Geometry: see drawing. Coordinates: mm, zero at the bounding-box minimum. A direction names the side the tool comes from. Round coordinates to 2 decimals unless told otherwise and drop trailing zeros. Write each loop counter-clockwise with the first axis right and the second up, starting at its lowest first coordinate (ties: lowest second). Pieces come first, ordered by that corner, then holes. Notation, with made-up numbers: (66, 80.5) -> (96, 80.5) arc R30 cw to (96, 108.5) -> close; hole circle Ø4 at (0, 56). An arc over 180 degrees is marked (long way). Write item = value, one per line.
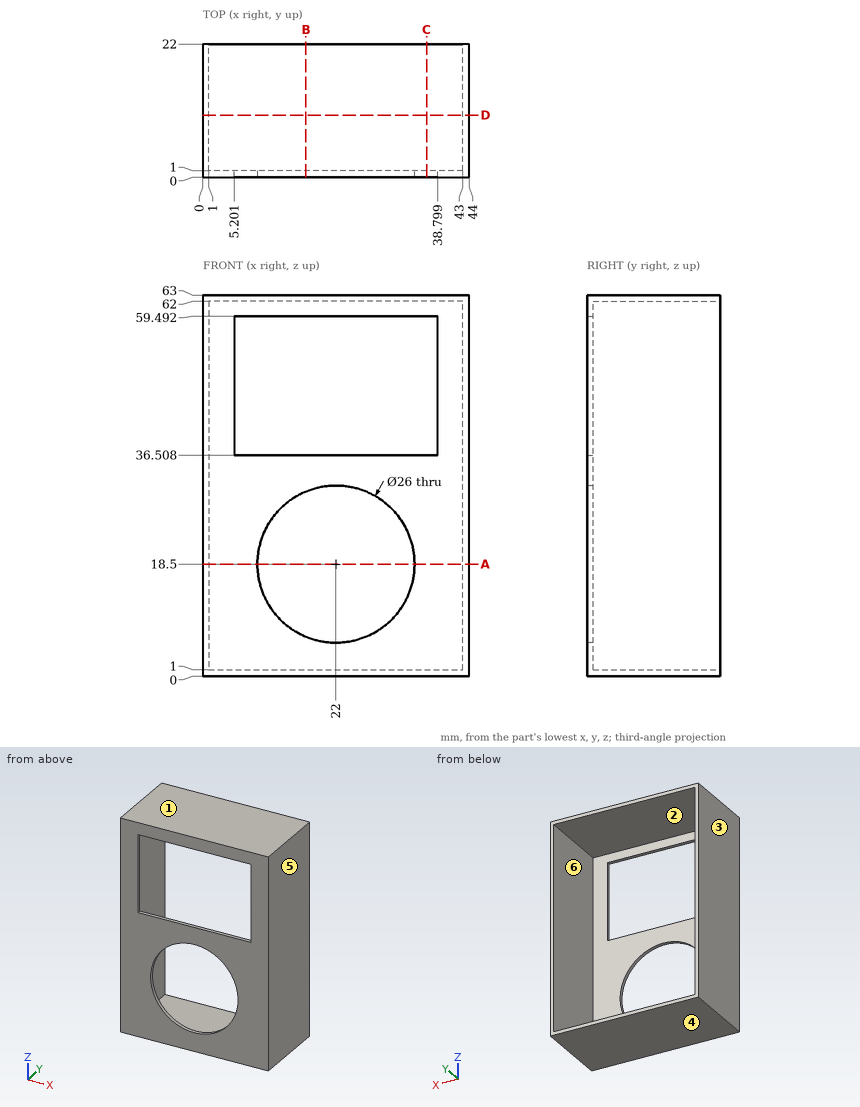
1) Cut plane A-A (z = 18.5). Return the cut outline in (x, y).
Solutions:
outline = (0, 0) -> (9, 0) -> (9, 1) -> (1, 1) -> (1, 22) -> (0, 22) -> close; (35, 0) -> (44, 0) -> (44, 22) -> (43, 22) -> (43, 1) -> (35, 1) -> close
2) Cut plane C-C (x = 37). Return the cut outline in (y, z).
Solutions:
outline = (0, 0) -> (22, 0) -> (22, 1) -> (1, 1) -> (1, 36.51) -> (0, 36.51) -> close; (0, 59.49) -> (1, 59.49) -> (1, 62) -> (22, 62) -> (22, 63) -> (0, 63) -> close
3) Line query: L1, parallel to Z at x = 22, y = 0.7; L2, parallel to Z at x = 13.5, y = 18; L3, parallel to X at y = 0.65, z = 18.5. Output: solid intervals per line, ascending. Write a range as from..to.
Solutions:
L1 = 0..5.5, 31.5..36.51, 59.49..63
L2 = 0..1, 62..63
L3 = 0..9, 35..44
4) Access query for the marked faces 1 and 2. Directions: +Z, -Z, +X, -X, +Y, -Y. A direction counts if a zero-diameter tool reaches every point of the face in a straight line with its end or side. Return the directions, or none.
Solutions:
face_1 = +Z, +X, -X, +Y, -Y
face_2 = +Y
5) Cut plane D-D (y = 10.25). Return the cut outline in (x, z).
Solutions:
outline = (0, 0) -> (44, 0) -> (44, 63) -> (0, 63) -> close; hole (1, 1) -> (43, 1) -> (43, 62) -> (1, 62) -> close
6) Draft query along X for the marked faces 3, 4, 5 and 6. Return one class per face: +X half, -X half, draft (parallel to the pull), parting line (faces both ways), or undercut.
Solutions:
face_3 = -X half
face_4 = draft
face_5 = +X half
face_6 = undercut
7) Cut plane B-B (x = 17). Return the cut outline in (y, z).
Solutions:
outline = (0, 0) -> (22, 0) -> (22, 1) -> (1, 1) -> (1, 6.5) -> (0, 6.5) -> close; (0, 30.5) -> (1, 30.5) -> (1, 36.51) -> (0, 36.51) -> close; (0, 59.49) -> (1, 59.49) -> (1, 62) -> (22, 62) -> (22, 63) -> (0, 63) -> close
8) First-contact query: P1, Ø10, axis at x = 22, z = 15, coming from the +Y side. Flat tip, straight axial feed; report the tip coordinate or a pass-through.
Solutions:
P1 = through
